```python
from build123d import *

# Parameters (mm, degrees)
ESQUISSE1_R                  = 14
ESQUISSE1_R_2                = 6
BOSS_EXTRU_1_DEPTH           = 7
ESQUISSE2_R                  = 14
ESQUISSE2_R_2                = 8
ENL_V_MAT_EXTRU_1_DEPTH      = 1
ESQUISSE3_OUTSIDE_W          = 38.042
ESQUISSE3_OUTSIDE_H          = 38.042
ESQUISSE3_OUTSIDE_R          = 8
ENL_V_MAT_EXTRU_2_DEPTH      = 3.5
ESQUISSE4_R                  = 1.3
ENL_V_MAT_EXTRU_3_DEPTH      = 8
R_P_TITION_CIRCULAIRE1_COUNT = 3


with BuildPart() as part:
    # Esquisse1 → Boss.-Extru.1 (new body)
    with BuildSketch(Plane.XY):
        Circle(ESQUISSE1_R)
        Circle(ESQUISSE1_R_2, mode=Mode.SUBTRACT)
    extrude(amount=BOSS_EXTRU_1_DEPTH)

    # Esquisse2 → Enlèv. mat.-Extru.1 (cut)
    with BuildSketch(Plane.XY.offset(7)):
        Circle(ESQUISSE2_R)
        Circle(ESQUISSE2_R_2, mode=Mode.SUBTRACT)
    extrude(amount=-ENL_V_MAT_EXTRU_1_DEPTH, mode=Mode.SUBTRACT)

    # Esquisse3 outside → Enlèv. mat.-Extru.2 (cut)
    with BuildSketch(Plane(origin=(0, 0, 0), x_dir=(-1, 0, 0), z_dir=(0, 0, -1))):
        Rectangle(ESQUISSE3_OUTSIDE_W, ESQUISSE3_OUTSIDE_H)
        Circle(ESQUISSE3_OUTSIDE_R, mode=Mode.SUBTRACT)
    extrude(amount=-ENL_V_MAT_EXTRU_2_DEPTH, mode=Mode.SUBTRACT)

    # Esquisse4 → Enlèv. mat.-Extru.3 (cut)
    with BuildSketch(Plane.XY):
        with Locations((0, 11)):
            Circle(ESQUISSE4_R)
    enl_v_mat_extru_3 = extrude(amount=ENL_V_MAT_EXTRU_3_DEPTH, mode=Mode.SUBTRACT)

    # Répétition circulaire1: Enlèv. mat.-Extru.3 ×3 about axis
    r_p_tition_circulaire1_axis = Axis((0, 0, 0), (0, 0, 1))
    for i in range(1, R_P_TITION_CIRCULAIRE1_COUNT):
        add(enl_v_mat_extru_3.rotate(r_p_tition_circulaire1_axis, i * 360 / R_P_TITION_CIRCULAIRE1_COUNT), mode=Mode.SUBTRACT)


solid = part.part
```
Work out the finished part from the listing and answer in its coordinate system (mm). A direction names the side the tool comes from. Give positions to 0.01 mm unless a question says otherwise; leave off trailing zeros. Order: outer loops, then holes, each group sorted by start corner. A loop starts at its lowest first (then second) coordinate and runs counter-clockwise, first axis right, second up. Notation, with made-up numbers: M 41,65.25 L 95,65.25 A32 cw 95,99.25 Z; hole C 16,-17 d8. An arc over 180 degrees is marked long. Return JSON: item names as keys, results as strings.
1) Each of these flat-tipped pins is pushed along its axis until it touches: pin 1 (3.5 mm diameter, centred on x = -9.53, y = -5.5, fed in from -Z); pin 2 (3 mm diameter, centred on x = 0, y = 11, fed in from +Z); pin 3 (2 mm diameter, centred on x = 9.53, y = -5.5, fed in from -Z). Where does it stop, or does it pass through?
Resolved:
{"pin 1": "z = 3.5", "pin 2": "z = 6", "pin 3": "through"}
2) Straight lines are drawn through the part: line 1 along Y through (x, z) = (0, 4.2); line 2 along Y through (x, z) = (0.5, 4.5); line 3 along Z through (x, y) = (10, 4.5). For each, find the intervals that lie inside material, in ascending order. Write a range as [from, to].
Resolved:
{"line 1": "[-14, -6], [6, 9.7], [12.3, 14]", "line 2": "[-13.99, -5.98], [5.98, 9.8], [12.2, 13.99]", "line 3": "[3.5, 6]"}
3) Section A-A, the plane x = 0 is taken. Write down the section's boundary in (y, z), plus the area to 3 significant figures.
Resolved:
{"outline": "M -14,3.5 L -8,3.5 L -8,0 L -6,0 L -6,7 L -8,7 L -8,6 L -14,6 Z; M 6,0 L 8,0 L 8,3.5 L 9.7,3.5 L 9.7,6 L 8,6 L 8,7 L 6,7 Z; M 12.3,3.5 L 14,3.5 L 14,6 L 12.3,6 Z", "area": "51.5 mm^2"}
4) Section C-C, the plane y = -5.5 is taken. Write down the section's boundary in (x, z).
Resolved:
{"outline": "M -12.87,3.5 L -10.83,3.5 L -10.83,6 L -12.87,6 Z; M -8.23,3.5 L -5.81,3.5 L -5.81,0 L -2.4,0 L -2.4,7 L -5.81,7 L -5.81,6 L -8.23,6 Z; M 2.4,0 L 5.81,0 L 5.81,3.5 L 8.23,3.5 L 8.23,6 L 5.81,6 L 5.81,7 L 2.4,7 Z; M 10.83,3.5 L 12.87,3.5 L 12.87,6 L 10.83,6 Z"}
5) A tool of negligible diameter and unlimited length cuts with its end or side. For faces 5 (the cylindrical face through (-1.73, -7.81, 6.51)), 6 (the cylindrical face through (1.73, -7.81, 1.73)), 7 (the flat face through (-2, 6, 0)), from which of +Z, -Z, +X, -X, +Y, -Y can it reach the whole face along a straight path? Write none if from no direction.
Resolved:
{"face 5": "+Z", "face 6": "-Z", "face 7": "-Z, +X, -X, +Y, -Y"}
6) Section D-D, the plane z = 3 is taken. Write down the section's boundary in (x, y).
Resolved:
{"outline": "C 0,0 d16; hole C 0,0 d12"}
7) For a pull along Y with two mould halves and no side action, classify faces 1 (the cylindrical face through (-6, 0, 3)), 2 (the cylindrical face through (12.932, -5.362, 4.732)), 3 (the flat face through (-6, -6, 3.5)), 4 (the cylindrical face through (-8.325, -5.998, 4.732)) as +Y half, -Y half, draft (parallel to the pull), parting line (faces both ways), or undercut.
Resolved:
{"face 1": "undercut", "face 2": "parting line", "face 3": "draft", "face 4": "undercut"}
8) Section B-B, the plane y = 0 is taken. Write down the section's boundary in (x, z), plus the area to 3 significant figures.
Resolved:
{"outline": "M -14,3.5 L -8,3.5 L -8,0 L -6,0 L -6,7 L -8,7 L -8,6 L -14,6 Z; M 6,0 L 8,0 L 8,3.5 L 14,3.5 L 14,6 L 8,6 L 8,7 L 6,7 Z", "area": "58.0 mm^2"}
